Geometry check sheet. Reference: drawing and pictorial views, mm from the part's lowest x, y, z. A direction names the side the tool comes from. Give positions to 0.01 mm unless a question says otherwise; leave off trailing zeros. Write each loop counter-clockwise with the first axis right and the second up, starting at its lowest first coordinate (ties: lowest second). Pieces come first, ordered by that corner, then holes. Notation, with made-up numbers: (86.25, 52) -> (137.25, 52) arc R18 cw to (137.25, 71) -> close; hole circle Ø6 at (60, 23). An arc over 180 degrees is marked (long way). Use a Markdown table: item, result. Add a question column.
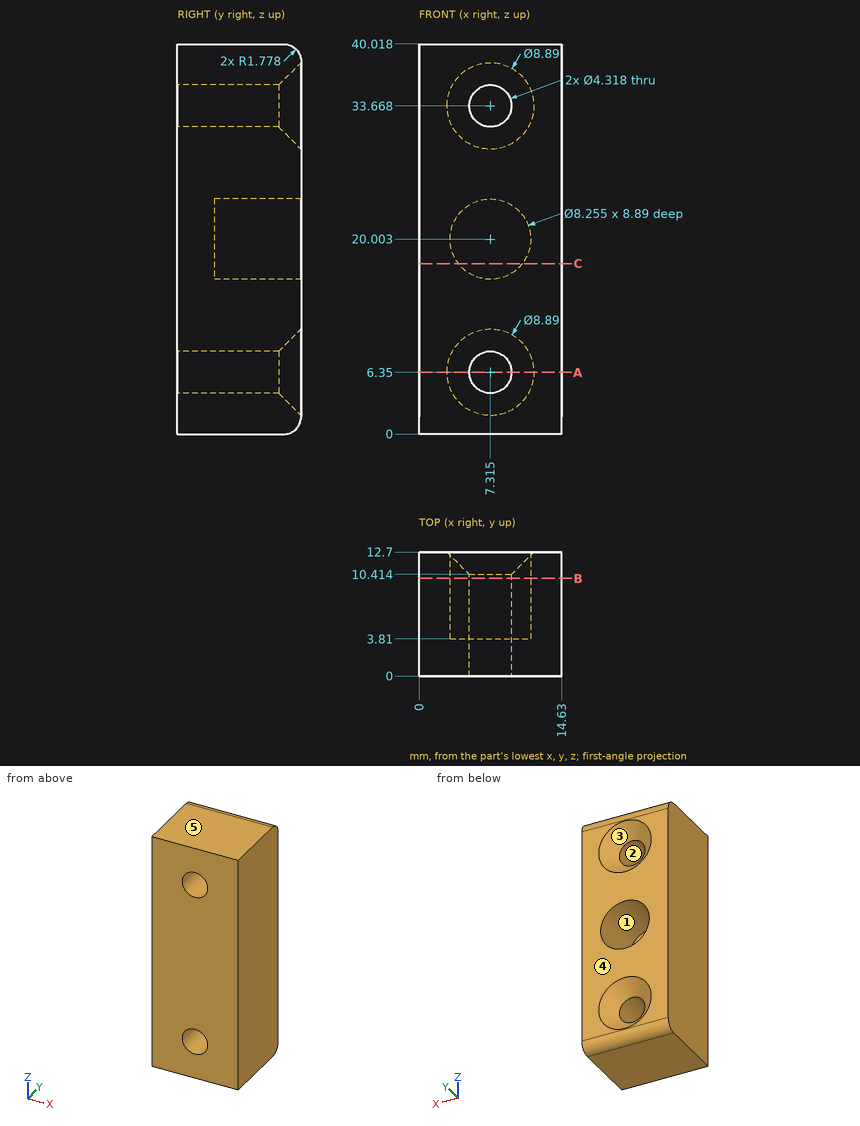
1) Sectioned sample at A-A, the plane z = 6.35. Enter the section's corners in (x, y) (1 decimal).
2) Draft check along Z on the marked faces 3, 4 and 5. Enter one of: +Z half, -Z half, draft (parallel to the pull), parting line (faces both ways), or undercut.
3) Sectioned sample at B-B, the plane y = 10. Count the separate pieces of the cut face and the enclosed holes in it, and give its area (3 significant figures).
4) Gauge pin test, flat ends, axial feed: P1, Ø2.5, axis at x = 8.5, z = 21.5, coming from the +Y side; P2, Ø2, axis at x = 8, y = 8, coming from the -Z side. Record the tip position at first contact, or that the pin passes through.
5) Tool access check on the marked faces 1 and 2. Record the directions out of +Z, -Z, +X, -X, +Y, -Y that give a thin tool (end or side, any length) a straight path to the whole face; none if there is none.
6) Material ranges on probe 1 along Z at (x, y) = (7.75, 4) (1 decimal); probe 2 along Z at (x, y) = (8.75, 4.75) (1 decimal); probe 3 along X at (y, z) = (5.5, 16.5) (1 decimal), recorded low to high. Write a range as [from, to].
7) Sectioned sample at C-C, the plane z = 17.5. Enter the section's corners in (x, y).
Check values:
| question | item | result |
|---|---|---|
| 1 | outline | (0, 0) -> (5.2, 0) -> (5.2, 10.4) -> (2.9, 12.7) -> (0, 12.7) -> close; (9.5, 0) -> (14.6, 0) -> (14.6, 12.7) -> (11.8, 12.7) -> (9.5, 10.4) -> close |
| 2 | face 3 | undercut |
| 2 | face 4 | draft |
| 2 | face 5 | +Z half |
| 3 | separate pieces | 1 |
| 3 | enclosed holes | 3 |
| 3 | area | 503 mm² |
| 4 | P1 | y = 3.81 |
| 4 | P2 | z = 0 |
| 5 | face 1 | +Y |
| 5 | face 2 | +Y, -Y |
| 6 | probe 1 | [0, 4.2], [8.5, 15.9], [24.1, 31.6], [35.8, 40] |
| 6 | probe 2 | [0, 4.7], [8, 16.1], [23.9, 32.1], [35.3, 40] |
| 6 | probe 3 | [0, 5.1], [9.5, 14.6] |
| 7 | outline | (0, 0) -> (14.63, 0) -> (14.63, 12.7) -> (10.6, 12.7) -> (10.6, 3.81) -> (4.03, 3.81) -> (4.03, 12.7) -> (0, 12.7) -> close |
